CAD build for the part. Positions are in the model's coordinates, mm. Coordinates: 2 decimals unless noted, no trailing zeros. Loops run counter-clockwise (first coordinate to the right, second up) from the corner with the lowest first, then second, coordinate; pieces in that order, holes last. Notation, with made-up numbers: (11, 14.5) - (20, 14.5) arc R14 cw to (20, 26.5) - close; hole circle Ø2 at (-24.75, 73). An arc over 180 degrees is marked (long way). Put each result on its own line as item: value.
```python
from build123d import *

# Parameters (mm, degrees)
SKETCH_1_R      = 3
EXTRUDE_1_DEPTH = 7
SKETCH_2_R      = 0.25
EXTRUDE_2_DEPTH = 3
FILLET_1_R      = 0.5


with BuildPart() as part:
    # Эскиз1 → Вытянуть1 (new body)
    with BuildSketch(Plane.XY):
        Circle(SKETCH_1_R)
    extrude(amount=EXTRUDE_1_DEPTH)

    # Эскиз2 → Вытянуть2 (add)
    with BuildSketch(Plane(origin=(0, 0, 0), x_dir=(-1, 0, 0), z_dir=(0, 0, -1))):
        with Locations(Location((-1.25, 0, 0), (0, 0, 180))):
            Circle(SKETCH_2_R)
        with Locations(Location((1.25, 0, 0), (0, 0, 180))):
            Circle(SKETCH_2_R)
    extrude(amount=EXTRUDE_2_DEPTH)

    # Скругление1
    fillet_1_edges = [part.edges().sort_by_distance(p)[0] for p in [
        (-3, 0, 7),
    ]]
    fillet(fillet_1_edges, radius=FILLET_1_R)


solid = part.part
```
Q1. Slice it at A-A, the plane y = 0. Give the cut face in (x, z).
Determined:
outline: (-3, 0) - (-1.5, 0) - (-1.5, -3) - (-1, -3) - (-1, 0) - (1, 0) - (1, -3) - (1.5, -3) - (1.5, 0) - (3, 0) - (3, 6.5) arc R0.5 ccw to (2.5, 7) - (-2.5, 7) arc R0.5 ccw to (-3, 6.5) - close
Q2. Slice it at B-B, the plane z = -2.5. Give the cut face in (x, y).
Determined:
outline: circle Ø0.5 at (-1.25, 0); circle Ø0.5 at (1.25, 0)
Q3. Pin check, flat tip, straight feed: pin 1 Ø2 at (y, z) = (2, 3.5) entering from +X. Stop position of the tip, or through.
Determined:
pin 1: x = 2.83
Q4. Wall check: L1, parallel to Z at x = 1, y = 0.3; L2, parallel to Y at x = 1.25, z = -0.75; L3, parallel to Y at x = 0.5, z = 4. Give the ranges that are in metal, low to high. Write a range as from..to.
Determined:
L1: 0..7
L2: -0.25..0.25
L3: -2.96..2.96
Q5. Slice it at D-D, the plane z = 0.25. Give the cut face in (x, y).
Determined:
outline: circle Ø6 at (0, 0)
Q6. Slice it at C-C, the plane x = 0. Give the cut face in (y, z), then the cut area to 3 significant figures.
Determined:
outline: (-3, 0) - (3, 0) - (3, 6.5) arc R0.5 ccw to (2.5, 7) - (-2.5, 7) arc R0.5 ccw to (-3, 6.5) - close
area: 41.9 mm2
